Read the model definition and answer for the solid it produces. Units are mm, in the model's axes. A direction names the side the tool comes from. Round coordinates to 2 decimals unless told otherwise and drop trailing zeros. Write each loop counter-clockwise with the first axis right and the second up, starting at its lowest first coordinate (ties: lowest second). Pieces come first, ordered by that corner, then holes. Notation, with made-up numbers: (-17, 11.5) - (33, 11.5) arc R22 ccw to (33, 24.5) - close; hole circle Ø7 at (54, -25.75). An arc over 180 degrees is marked (long way). Answer as CSV lines item,"result". Start each with the question number.
1) Which of the six approach directions +Z, -Z, +X, -X, +Y, -Y give full straight-line access (tool end or side, diameter ignored) to faces 4 (the cylindrical face through (-1.92, 3.395, 14.857)), 5 (the cylindrical face through (-1.92, 3.395, 0.143)), 6 (the flat face through (-1.901, 3.232, 7.402)), 7 (the flat face through (-6, -1, 6))?
2) Consider line 1 along Z through (x, y) = (-9.8, 0); line 2 along Z through (x, y) = (-5, -3.5); line 3 along X through (y, z) = (4.75, 8.5). Determine where each line is inside the solid, lowest interval first.
3) Find section B-B on z = 8. State how many separate pieces and enclosed holes the cut face has, then the cut area to 3 significant figures.
4) Find section C-C on x = 5.5. Determine the outline of the cut face in (y, z), then the cut area to 3 significant figures.
5) For a pull along Z with two mould halves and no side action, classify faces 1 (the flat face through (-5, -1, 13)), 2 (the flat face through (1.901, -3.232, 7.402)), 3 (the cylindrical face through (1.98, 3.361, 0.143)) as +Z half, -Z half, draft (parallel to the pull), parting line (faces both ways), or undercut.
6) Find section A-A on y = 0. Determine the outline of the cut face in (x, z).
from build123d import *

# Parameters (mm, degrees)
F0_W          = 20
F0_H          = 14
F1_DEPTH      = 15
F2_W          = 2.39
F2_H          = 11
F3_DEPTH      = 14.001
F5_R          = 0.5
F4_R          = 1.75
F6_DEPTH      = 42
F6_DEPTH_BACK = 20.001


# Not quite as in the source:
# - an extrude ends at something that could not be found from the text; its depth is read off the source's solid


with BuildPart() as f1:
    # F0 (on Top) → F1 (new body)
    with BuildSketch(Plane.XY):
        with Locations((-1, -0.4900455125)):
            Rectangle(F0_W, F0_H)
        Polygon((3.75, -2.1650635095), (0, -4.3301270189), (-3.75, -2.1650635095), (-3.75, 2.1650635095), (0, 4.3301270189), (3.75, 2.1650635095), align=None, mode=Mode.SUBTRACT)
    extrude(amount=F1_DEPTH)

    # F2 (on face) → F3 (cut, through all)
    with BuildSketch(Plane.XZ.offset(7.4900455125)):
        with Locations((-4.805, 7.5)):
            Rectangle(F2_W, F2_H)
    extrude(amount=-F3_DEPTH, mode=Mode.SUBTRACT)

    # F5
    f5_edges = [f1.edges().sort_by_distance(p)[0] for p in [
        (-11, -7.490046, 7.5),
        (-1, -7.490046, 0),
        (-1, -7.490046, 15),
        (9, -7.490046, 7.5),
        (-3.61, -7.490046, 7.5),
        (-4.805, -7.490046, 2),
        (-6, -7.490046, 7.5),
        (-4.805, -7.490046, 13),
        (9, 6.509954, 7.5),
        (-1, 6.509954, 0),
        (-1, 6.509954, 15),
        (-11, 6.509954, 7.5),
        (-4.805, 6.509954, 13),
        (-6, 6.509954, 7.5),
        (-4.805, 6.509954, 2),
        (-3.61, 6.509954, 7.5),
        (9, -0.490046, 15),
        (-11, -0.490046, 15),
        (3.75, 0, 15),
        (1.875, -3.247595, 15),
        (-1.875, -3.247595, 15),
        (-3.75, 0, 15),
        (-1.875, 3.247595, 15),
        (1.875, 3.247595, 15),
        (9, -0.490046, 0),
        (-11, -0.490046, 0),
        (3.75, 0, 0),
        (1.875, -3.247595, 0),
        (-1.875, -3.247595, 0),
        (-3.75, 0, 0),
        (-1.875, 3.247595, 0),
        (1.875, 3.247595, 0),
    ]]
    fillet(f5_edges, radius=F5_R)

    # F4 (on face) → F6 (cut, two sides)
    with BuildSketch(Plane(origin=(-11, 0, 0), x_dir=(0, -1, 0), z_dir=(-1, 0, 0))) as f6_sk:
        with Locations((0, 8)):
            Circle(F4_R)
    extrude(amount=F6_DEPTH, mode=Mode.SUBTRACT)
    extrude(f6_sk.sketch, amount=-F6_DEPTH_BACK, mode=Mode.SUBTRACT)


solid = f1.part
Check values:
1,face 4,"+Z"
1,face 5,"-Z"
1,face 6,"+Z, -Z"
1,face 7,"+Y, -Y"
2,line 1,"z = 0 to 6.25, 9.75 to 15"
2,line 2,"z = 0 to 2, 13 to 15"
2,line 3,"x = -11 to -6, -3.61 to 9"
3,separate pieces,"4"
3,enclosed holes,"0"
3,area,"162 mm^2"
4,outline,"(-7.49, 0.5) arc R0.5 ccw to (-6.99, 0) - (6.01, 0) arc R0.5 ccw to (6.51, 0.5) - (6.51, 14.5) arc R0.5 ccw to (6.01, 15) - (-6.99, 15) arc R0.5 ccw to (-7.49, 14.5) - close; hole circle Ø3.5 at (0, 8)"
4,area,"200 mm^2"
5,face 1,"undercut"
5,face 2,"draft"
5,face 3,"-Z half"
6,outline,"(-11, 0.5) arc R0.5 ccw to (-10.5, 0) - (-4.25, 0) arc R0.5 ccw to (-3.75, 0.5) - (-3.75, 2) - (-6, 2) - (-6, 6.25) - (-11, 6.25) - close; (-11, 9.75) - (-6, 9.75) - (-6, 13) - (-3.75, 13) - (-3.75, 14.5) arc R0.5 ccw to (-4.25, 15) - (-10.5, 15) arc R0.5 ccw to (-11, 14.5) - close; (3.75, 0.5) arc R0.5 ccw to (4.25, 0) - (8.5, 0) arc R0.5 ccw to (9, 0.5) - (9, 6.25) - (3.75, 6.25) - close; (3.75, 9.75) - (9, 9.75) - (9, 14.5) arc R0.5 ccw to (8.5, 15) - (4.25, 15) arc R0.5 ccw to (3.75, 14.5) - close"
